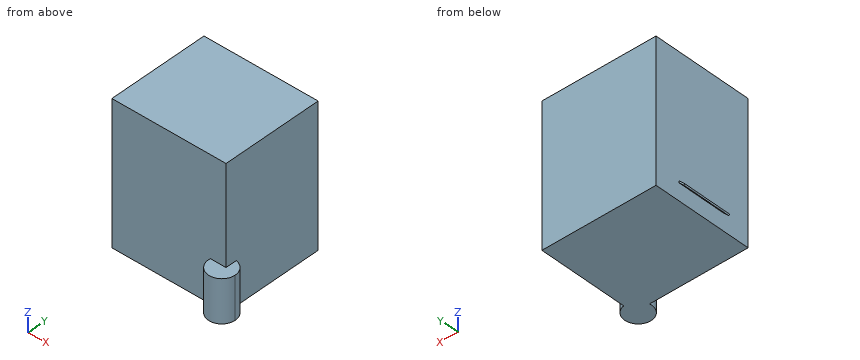
```python
from build123d import *

# Parameters (mm, degrees)
F1_DEPTH      = 330
F2_DEPTH      = 100
F4_DEPTH      = 72.5
F4_DEPTH_BACK = 42.5


with BuildPart() as f1:
    # F0 (on Top) → F1 (new body)
    with BuildSketch(Plane.XY):
        with BuildLine():
            Line((-137, 101), (-137, -135))
            Line((-137, -135), (94.248996, -135))
            ThreePointArc((94.248996, -135), (107.058017, -114.066985), (131, -108.677774))
            Line((131, -108.677774), (131, 101))
            Line((131, 101), (-137, 101))
        make_face()
        with BuildLine():
            ThreePointArc((131, -108.677774), (107.058017, -114.066985), (94.248996, -135))
            Line((94.248996, -135), (131, -135))
            Line((131, -135), (131, -108.677774))
        make_face()
    extrude(amount=F1_DEPTH)

    # F0 (on Top) → F2 (join)
    with BuildSketch(Plane.XY):
        with BuildLine():
            Line((131, -135), (94.248996, -135))
            ThreePointArc((94.248996, -135), (123.055497, -171.08863), (156.9, -139.676))
            ThreePointArc((156.9, -139.676), (149.572815, -119.478847), (131, -108.677774))
            Line((131, -108.677774), (131, -135))
        make_face()
    extrude(amount=F2_DEPTH)

    # F3 (on Front) → F4 (join, two sides)
    with BuildSketch(Plane.XZ) as f4_sk:
        Polygon((-137, 44.192641), (-151.07132, 30.12132), (-148.95, 28), (-134.87868, 42.07132), align=None)
    extrude(amount=F4_DEPTH)
    extrude(f4_sk.sketch, amount=-F4_DEPTH_BACK)


solid = f1.part
```
The listing builds one solid part. Answer for the finished solid, in the listing's coordinates (mm). Coordinates: 2 decimals unless noted, no trailing zeros. Write each loop counter-clockwise with the first axis right and the second up, starting at its lowest first coordinate (ties: lowest second). Pieces come first, ordered by that corner, then holes. Notation, with made-up numbers: M -34,-35 L -27,-35 A23 cw -27,-19 Z; hole C 33,-36.5 d10. An arc over 180 degrees is marked long. Use a Markdown table: item, result. Add a question column.
1. Section A-A (x = 125.4) is taken. Give the vertices of the cut face in (y, z).
2. Given P1, Ø4, axis at x = -144, z = 36, coming from the +Y side; P2, Ø3, axis at y = 30, z = 95.5, coming from the +X side; P3, Ø4, axis at y = -130.5, z = 35.5, coming from the +X side; P4, Ø18.5, axis at x = 139, y = -132.5, coming from the +Z side, each flat-ended and moving along its own axis, determine where each tip first touches the part or whether it passes through.
3. Section D-D (x = 32) is taken. Give the vertices of the cut face in (y, z).
4. Section B-B (y = -37.5) is taken. Give the vertices of the cut face in (x, z), plus the area to 3 significant figures.
5. Straight lines are drawn through the part: line 1 along X through (y, z) = (-66, 16); line 2 along Y through (x, z) = (-30.5, 313); line 3 along Z through (x, y) = (133.5, -144). For each, find the intervals that lie inside material, in ascending order. Write a range as [from, to].
6. Section C-C (z = 270.5) is taken. Give the vertices of the cut face in (x, y), plus the area to 3 significant figures.
Data:
| question | item | result |
|---|---|---|
| 1 | outline | M -171.18,0 L 101,0 L 101,330 L -135,330 L -135,100 L -171.18,100 Z |
| 2 | P1 | stops at y = 42.5 |
| 2 | P2 | stops at x = 131 |
| 2 | P3 | stops at x = 156.07 |
| 2 | P4 | stops at z = 330 |
| 3 | outline | M -135,0 L 101,0 L 101,330 L -135,330 Z |
| 4 | outline | M -151.07,30.12 L -148.95,28 L -137,39.95 L -137,0 L 131,0 L 131,330 L -137,330 L -137,44.19 Z |
| 4 | area | 88,500 mm2 |
| 5 | line 1 | x = [-137, 131] |
| 5 | line 2 | y = [-135, 101] |
| 5 | line 3 | z = [0, 100] |
| 6 | outline | M -137,-135 L 131,-135 L 131,101 L -137,101 Z |
| 6 | area | 63,200 mm2 |
